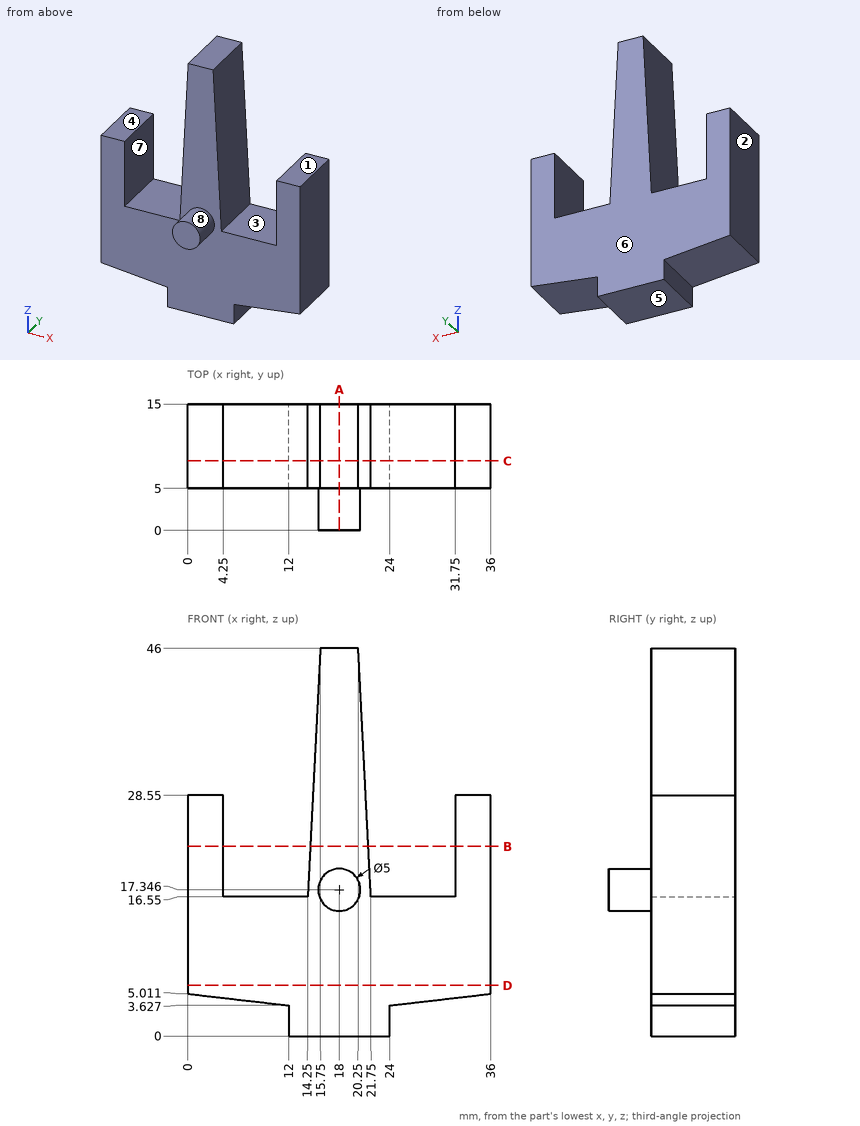
Geometry check sheet. Reference: drawing and pictorial views, mm from the part's lowest x, y, z. A direction names the side the tool comes from. Coordinates: 2 decimals unless noted, no trailing zeros. Order: outer loops, then holes, each group sorted by start corner. A loop starts at its lowest first (then second) coordinate and runs counter-clockwise, first axis right, second up. Notation, with made-up numbers: (-19, -37.5) -> (13, -37.5) arc R17 ccw to (13, -6.5) -> close; hole circle Ø3 at (54.5, 69). An arc over 180 degrees is marked (long way). Use CSV: the item, a comma, the result in double quotes. Start each with the question number.
Q1. Section check C-C, the plane y = 8.25. Record the cut outline in (x, z), and give its area (3 significant figures).
Q2. Section check D-D, the plane z = 6. Record the cut outline in (x, y), and give its area (3 significant figures).
Q3. Thickness scan on line 1 along X through (y, z) = (14.75, 20.5); line 2 along Z through (x, y) = (22, 8); line 3 along Y through (x, z) = (12.5, 6). Record the ranges inside material, lowest first.
Q4. Draft check along X on the marked faces 6, 7 and 8. Enter one of: +X half, -X half, draft (parallel to the pull), parting line (faces both ways), or undercut.
Q5. Section check B-B, the plane z = 22.5. Record the cut outline in (x, y).
Q6. Depth check by flat-ended pin: P1, Ø5, axis at x = 28, y = 10.5, coming from the +Z side; P2, Ø1.3, axis at x = 34.5, y = 10.5, coming from the +Z side; P3, Ø1.8, axis at y = 9, z = 2, coming from the +X side. Enter the tip coordinate at first touch or a pass-through.
Q7. Section check A-A, the plane x = 18. Record the cut outline in (y, z).
Q8. Tool access check on the marked faces 1, 2, 3, 4 and 5. Record the directions out of +Z, -Z, +X, -X, +Y, -Y that give a thin tool (end or side, any length) a straight path to the whole face; none if there is none.
Returned:
1,outline,"(0, 5.01) -> (12, 3.63) -> (12, 0) -> (24, 0) -> (24, 3.63) -> (36, 5.01) -> (36, 28.55) -> (31.75, 28.55) -> (31.75, 16.55) -> (21.75, 16.55) -> (20.25, 46) -> (15.75, 46) -> (14.25, 16.55) -> (4.25, 16.55) -> (4.25, 28.55) -> (0, 28.55) -> close"
1,area,"771 mm^2"
2,outline,"(0, 5) -> (36, 5) -> (36, 15) -> (0, 15) -> close"
2,area,"360 mm^2"
3,line 1,"x = 0 to 4.25, 14.45 to 21.55, 31.75 to 36"
3,line 2,"z = 0 to 16.55"
3,line 3,"y = 5 to 15"
4,face 6,"draft"
4,face 7,"undercut"
4,face 8,"parting line"
5,outline,"(0, 5) -> (4.25, 5) -> (4.25, 15) -> (0, 15) -> close; (14.55, 5) -> (21.45, 5) -> (21.45, 15) -> (14.55, 15) -> close; (31.75, 5) -> (36, 5) -> (36, 15) -> (31.75, 15) -> close"
6,P1,"stops at z = 16.55"
6,P2,"stops at z = 28.55"
6,P3,"stops at x = 24"
7,outline,"(0, 14.85) -> (5, 14.85) -> (5, 0) -> (15, 0) -> (15, 46) -> (5, 46) -> (5, 19.85) -> (0, 19.85) -> close"
8,face 1,"+Z, +X, +Y, -Y"
8,face 2,"+Z, -Z, -X, +Y, -Y"
8,face 3,"+Z, +Y, -Y"
8,face 4,"+Z, -X, +Y, -Y"
8,face 5,"-Z, +X, -X, +Y, -Y"
